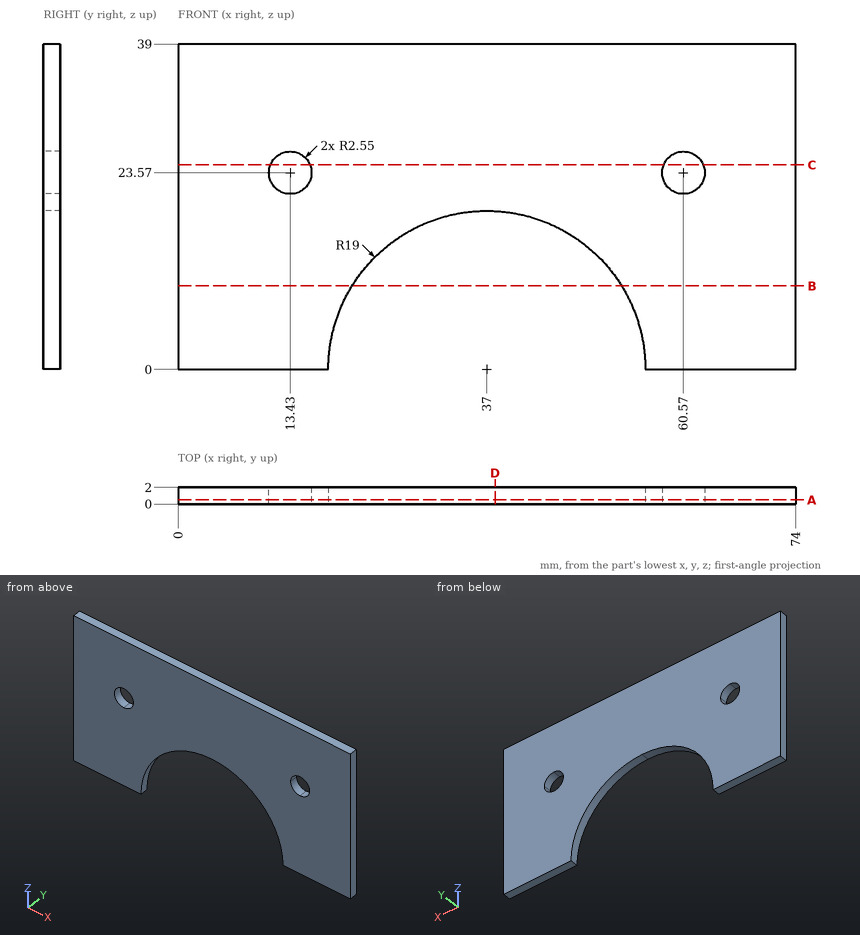
Geometry check sheet. Reference: drawing and pictorial views, mm from the part's lowest x, y, z. Coordinates: 2 decimals unless noted, no trailing zeros. Order: outer loops, then holes, each group sorted by start corner. A loop starts at its lowest first (then second) coordinate and runs counter-clockwise, first axis right, second up. Notation, with made-up numbers: M 89,-5.75 L 143,-5.75 A14 cw 143,17.25 Z; hole C 68,5 d9. An arc over 180 degrees is marked long. Return JSON: item names as keys, results as strings.
1) Cross-section at D-D, the plane x = 38. Record the boundary of the cut face in (y, z).
Answer list:
{"outline": "M 0,18.97 L 2,18.97 L 2,39 L 0,39 Z"}
2) Gauge pin test, flat ends, axial feed: pin 1 (1 mm diameter, centred on x = 17.5, z = 27.5, fed in from -Y); pin 2 (1.5 mm diameter, centred on x = 41.5, z = 16.5, fed in from +Y). Record the tip position at first contact, or that the pin passes through.
Answer list:
{"pin 1": "y = 0", "pin 2": "through"}
3) Cross-section at A-A, the plane y = 0.5. Record the boundary of the cut face in (x, z).
Answer list:
{"outline": "M 0,0 L 18,0 A19 cw 37,19 A19 cw 56,0 L 74,0 L 74,39 L 0,39 Z; hole M 13.43,21.02 A2.55 ccw 15.98,23.57 A2.55 ccw long Z; hole M 58.02,23.57 A2.55 ccw 60.57,21.02 A2.55 ccw 63.12,23.57 A2.55 ccw 60.57,26.12 A2.55 ccw Z"}
4) Cross-section at C-C, the plane z = 24.5. Record the boundary of the cut face in (x, y).
Answer list:
{"outline": "M 0,0 L 11.06,0 L 11.06,2 L 0,2 Z; M 15.8,0 L 58.2,0 L 58.2,2 L 15.8,2 Z; M 62.94,0 L 74,0 L 74,2 L 62.94,2 Z"}
5) Thickness scan on L1, parallel to X at y = 0.75, z = 23; L2, parallel to X at y = 1.25, z = 7.5; L3, parallel to X at y = 0.35, z = 5.5. Record the ranges inside material, lowest first. Write a range as [from, to].
Answer list:
{"L1": "[0, 10.94], [15.92, 58.08], [63.06, 74]", "L2": "[0, 19.54], [54.46, 74]", "L3": "[0, 18.81], [55.19, 74]"}
6) Cross-section at B-B, the plane z = 10. Record the boundary of the cut face in (x, y).
Answer list:
{"outline": "M 0,0 L 20.84,0 L 20.84,2 L 0,2 Z; M 53.16,0 L 74,0 L 74,2 L 53.16,2 Z"}
